Work out the finished part from the listing and answer in its coordinate system (mm). A direction names the side the tool comes from. Round coordinates to 2 decimals unless told otherwise and drop trailing zeros. Order: outer loops, then holes, each group sorted by start corner. A loop starts at its lowest first (then second) coordinate and runs counter-clockwise, first axis right, second up. Notation, with made-up numbers: (23.5, 83) - (61.5, 83) arc R27 cw to (61.5, 120) - close; hole circle Ø11 at (-9.75, 6.5). An arc over 180 degrees is marked (long way). Use CSV: the item, a comma, the result in double quotes.
Autodesk Inventor part; units mm, degrees
ref_plane "Work Plane1" through (12.7, 111.125, 12.7) normal (1, 0, 0) x (0, 0, -1)
ref_plane "YZ Plane" through (0, 0, 0) normal (1, 0, 0) x (0, 1, 0)
ref_plane "XZ Plane" through (0, 0, 0) normal (0, 1, 0) x (-1, 0, 0)
sketch "Sketch1" plane through (0, 0, 0) normal (0, 0, 1) x (1, 0, 0)
  line L0 (0, 0) -> (25.4, 0)
  line L1 (25.4, 0) -> (25.4, 111.125)
  line L2 (25.4, 111.125) -> (0, 111.125)
  line L3 (0, 111.125) -> (0, 0)
  dimension "d0" = 25.4
  dimension "d1" = 111.125
extrude "Extrusion1" add sketch "Sketch1" along normal blind 12.7
sketch "Sketch2" plane through (0, 0, 12.7) normal (0, 0, 1) x (1, 0, 0)
  line L0 (25.4, 111.125) -> (0, 111.125)
  line L1 (25.4, 0) -> (25.4, 111.125)
  point P0 (0, 0)
  point P1 (12.7, 22.225)
  dimension "d4" = 88.9
  dimension "d5" = 25.4
  dimension "d6" = 12.7
hole "Hole1" at (12.7, 22.225, 12.7) direction (0, 0, -1) diameter 6.35 end through all
sketch "Sketch3" plane through (0, 0, 12.7) normal (0, 0, 1) x (1, 0, 0)
  circle A0 centre (12.7, 22.225) radius 3.175
  line L0 (0, 111.125) -> (0, 0)
  point P0 (12.7, 30.226)
  dimension "d14" = 8.001
  dimension "d15" = 12.7
hole "Hole2" at (12.7, 30.226, 12.7) direction (0, 0, -1) diameter 3.175 end through all
pattern_circular "Circular Pattern1" count 6 over 360 about axis through (12.7, 22.225, -101.9962) along (0, 0, 1) of "Hole2"
sketch "Sketch5" plane through (25.4, 0, 0) normal (1, 0, 0) x (0, 0, -1)
  line L0 (0, 0) -> (-12.7, 0)
  line L1 (-12.7, 12.6365) -> (-12.7, 15.8115)
  line L2 (0, 0) -> (-12.7, 0)
  line L3 (-12.7, 0) -> (-12.7, 12.7)
  line L4 (-12.7, 12.7) -> (0, 12.7)
  line L5 (0, 12.7) -> (0, 0)
  dimension "d26" = 12.7
extrude "Extrusion2" add sketch "Sketch5" along normal blind 25.4
ref_plane "Work Plane1" through (12.7, 111.125, 12.7) normal (1, 0, 0) x (0, 0, -1)
mirror "Mirror1" about plane through (12.7, 111.125, 12.7) normal (1, 0, 0) of "Extrusion2"
sketch "Sketch7" plane through (50.8, 0, 0) normal (0, -1, 0) x (1, 0, 0)
  line L0 (-76.2, 0) -> (0, 0)
  line L1 (0, 12.7) -> (0, 0)
  line L2 (0, 12.7) -> (-76.2, 12.7)
  line L3 (-76.2, 12.7) -> (-76.2, 0)
  point P0 (-50.8, 0)
  point P1 (-6.35, 6.35)
  point P2 (-69.85, 6.35)
  dimension "d29" = 12.7
  dimension "d30" = 6.35
  dimension "d31" = 6.35
  dimension "d32" = 6.35
  dimension "d33" = 6.35
hole "Hole3" at (44.45, 0, 6.35) at (-19.05, 0, 6.35) direction (0, 1, 0) diameter 2.6416 end through all
properties part number "Motor Block" material "Aluminum 6061"
(1) Find the intervals of material crossed by L1, parallel to X at y = 2.5, z = 6.35; L2, parallel to Y at x = 6, z = 6 (3 decimals); L3, parallel to X at y = 30, z = 10, in increasing order. Write a range as from..to.
Findings below:
L1,"x = -25.4..-20.37, -17.73..43.13, 45.77..50.8"
L2,"y = 0..16.654, 19.795..24.655, 27.796..111.125"
L3,"x = 0..11.13, 14.27..25.4"
(2) For faces 1 (the flat face through (25.4, 61, 6)), 2 (the cylindrical face through (18.22, 26.96, 6.26)), determine the directions among +Z, -Z, +X, -X, +Y, -Y from which every point of the face is accessible in a straight line to the end or side of a thin tool.
Findings below:
face 1,"+Z, -Z, +X, +Y"
face 2,"+Z, -Z"
(3) Find section D-D (x = -19.05). Determine the outline of the cut face in (y, z), and give its area (3 significant figures).
Findings below:
outline,"(0, 0) - (12.7, 0) - (12.7, 5.03) - (0, 5.03) - close; (0, 7.67) - (12.7, 7.67) - (12.7, 12.7) - (0, 12.7) - close"
area,"128 mm²"
(4) Each of these flat-tipped pins is pushed along its axis until it touches: pin 1 (1.5 mm diameter, centred on x = 35.5, z = 7.5, fed in from +Y); pin 2 (4 mm diameter, centred on y = 81, z = 6.5, fed in from -X). Where does it stop, or does it pass through?
Findings below:
pin 1,"stops at y = 12.7"
pin 2,"stops at x = 0"
(5) The mould has two halves that part along Z. Classify faces 3 (the flat face through (-13, 12.7, 6)), 4 (the flat face through (13, 44, 12.7)), 5 (the cylindrical face through (45.74, 6.44, 6.64)): released by +Z, released by -Z, zero draft, split by the parting line, or undercut.
Findings below:
face 3,"zero draft"
face 4,"released by +Z"
face 5,"undercut"
(6) Find section A-A (x = 12.7). State how many separate pieces and enclosed holes the cut face has, and give its area (3 significant figures).
Findings below:
separate pieces,"4"
enclosed holes,"0"
area,"1,250 mm²"
(7) Find section C-C (y = 22). Determine the outline of the cut face in (x, z).
Findings below:
outline,"(0, 0) - (9.53, 0) - (9.53, 12.7) - (0, 12.7) - close; (15.87, 0) - (25.4, 0) - (25.4, 12.7) - (15.87, 12.7) - close"
